```python
from build123d import *

# Parameters (mm, degrees)
CROQUIS6_W              = 375
CROQUIS6_H              = 33
SALIENTE_EXTRUIR4_DEPTH = 33
CROQUIS7_W              = 275
CROQUIS7_H              = 230
SALIENTE_EXTRUIR5_DEPTH = 75
CHAFL_N2_START          = 77.927326738
CHAFL_N2_OUTLINE_W      = 275
CHAFL_N2_OUTLINE_H      = 245
CHAFL_N2_DEPTH          = 68.072673262
VACIADO4_T              = -3.5


with BuildPart() as part:
    # Croquis6 → Saliente-Extruir4 (new body)
    with BuildSketch(Plane.XY):
        Rectangle(CROQUIS6_W, CROQUIS6_H)
    extrude(amount=SALIENTE_EXTRUIR4_DEPTH)

    # Croquis7 → Saliente-Extruir5 (add)
    with BuildSketch(Plane(origin=(0, 16.5, 0), x_dir=(1, 0, 0), z_dir=(0, 1, 0))):
        with Locations((6.494e-05, 82)):
            Rectangle(CROQUIS7_W, CROQUIS7_H)
    extrude(amount=SALIENTE_EXTRUIR5_DEPTH)

    # Chaflán2: read off the stored shape, not the designer's step
    # Chaflán2 outline → Chaflán2 (cut)
    with BuildSketch(Plane(origin=(0, 0, 0), x_dir=(1, 0, 0), z_dir=(0, 0.9566738804288585, -0.2911616157826961)).offset(CHAFL_N2_START)):
        with Locations((6.494e-05, 62.5)):
            Rectangle(CHAFL_N2_OUTLINE_W, CHAFL_N2_OUTLINE_H)
    extrude(amount=CHAFL_N2_DEPTH, mode=Mode.SUBTRACT)

    # Vaciado4
    vaciado4_openings = [part.faces().sort_by_distance(p)[0] for p in [
        (-187.5, 0, 16.5),
        (187.5, 0, 16.5),
    ]]
    offset(amount=VACIADO4_T, openings=vaciado4_openings, kind=Kind.INTERSECTION)


solid = part.part
```
Read the model definition and answer for the solid it produces. Units are mm, in the model's axes. A direction names the side the tool comes from. Coordinates: 2 decimals unless noted, no trailing zeros. Loops run counter-clockwise (first coordinate to the right, second up) from the corner with the lowest first, then second, coordinate; pieces in that order, holes last.
(1) The part is cut by section C-C (z = -21.5). Determine the outline of the cut face in (x, y).
Solution:
outline: (-137.5, 16.5) - (137.5, 16.5) - (137.5, 74.91) - (-137.5, 74.91) - close; hole (-134, 20) - (134, 20) - (134, 71.25) - (-134, 71.25) - close
(2) The part is cut by section D-D (z = 11.5). Determine the outline of the cut face in (x, y), and give its area (3 significant figures).
Solution:
outline: (-187.5, -16.5) - (187.5, -16.5) - (187.5, -13) - (-187.5, -13) - close; (-187.5, 13) - (-134, 13) - (-134, 81.3) - (134, 81.3) - (134, 13) - (187.5, 13) - (187.5, 16.5) - (137.5, 16.5) - (137.5, 84.96) - (-137.5, 84.96) - (-137.5, 16.5) - (-187.5, 16.5) - close
area: 3,150 mm2
(3) The part is cut by section B-B (x = 86.5). Determine the outline of the cut face in (y, z), and give its area (3 significant figures).
Solution:
outline: (-16.5, 0) - (16.5, 0) - (16.5, -197) - (21.5, -197) - (91.5, 33) - (-16.5, 33) - close; hole (-13, 3.5) - (20, 3.5) - (20, -189.91) - (86.78, 29.5) - (-13, 29.5) - close
area: 2,110 mm2
(4) The mould has two halves that part along Y. Classify faces 4 (the face through (-3, 37, 33)), 5 (the face through (162, 16.5, 16)), 6 (the face through (134, 41, -30)): released by +Y, released by -Y, zero draft, split by the parting line, or undercut.
Solution:
face 4: zero draft
face 5: released by +Y
face 6: undercut
(5) Flat-ended cylindrical pins translate along their axes: pin 1 Ø5 at (x, y) = (88.5, 7.5) entering from -Z; pin 2 Ø3 at (x, z) = (-89.5, -91.5) entering from +Y; pin 3 Ø10 at (y, z) = (51, -8.5) entering from -X; pin 4 Ø12 at (y, z) = (7, -169.5) entering from -X. Find the tip coordinate at first contact, or state that the pin passes through.
Solution:
pin 1: stops at z = 0
pin 2: stops at y = 54.07
pin 3: stops at x = -137.5
pin 4: passes through
(6) The part is cut by section A-A (y = -9). Determine the outline of the cut face in (x, z).
Solution:
outline: (-187.5, 0) - (187.5, 0) - (187.5, 3.5) - (-187.5, 3.5) - close; (-187.5, 29.5) - (187.5, 29.5) - (187.5, 33) - (-187.5, 33) - close
(7) Consider line 1 along Z through (x, y) = (-42, 0); line 2 along X through (y, z) = (22, -174); line 3 along Y through (x, z) = (-19, 10). Determine where each line is inside the solid, lowest interval first.
Solution:
line 1: z = 0 to 3.5, 29.5 to 33
line 2: x = -137.5 to -134, 134 to 137.5
line 3: y = -16.5 to -13, 80.84 to 84.5
(8) A tool of negligible diameter and unlimited length cuts with its end or side. For faces 1 (the face through (-161, 13, 16)), 2 (the face through (-163, 16.5, 16)), 3 (the face through (-2, 16.5, -100)), from which of +Z, -Z, +X, -X, +Y, -Y can it reach the whole face along a straight path? Write none if from no direction.
Solution:
face 1: +X, -X
face 2: +Z, -Z, -X, +Y
face 3: -Z, +X, -X, -Y
